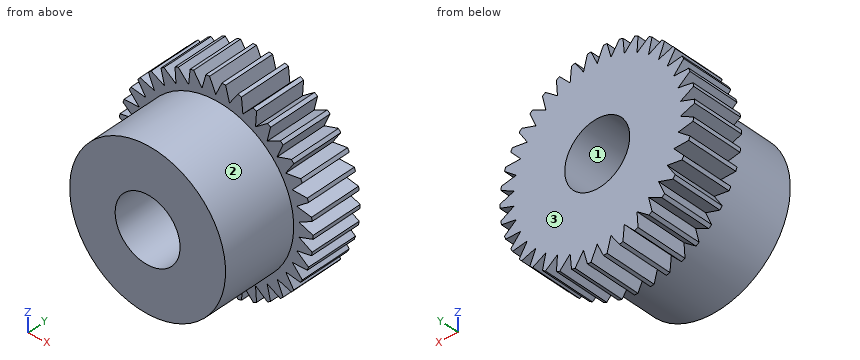
```python
from build123d import *

# Parameters (mm, degrees)
SKETCH_1_R          = 6
EXTRUDE_1_DEPTH     = 5.8
SKETCH_2_R          = 7.5
EXTRUDE_2_DEPTH     = 4
CUT_EXTRUDE_3_DEPTH = 15.440914098
SKETCH_4_R          = 2.5
CUT_EXTRUDE_4_DEPTH = 15.43297622


with BuildPart() as part:
    # Эскиз1 → Вытянуть1 (new body)
    with BuildSketch(Plane(origin=(0, 0, 0), x_dir=(1, 0, 0), z_dir=(0, 1, 0))):
        with Locations(Location((0, 0, 0), (0, 0, 270))):
            Circle(SKETCH_1_R)
    extrude(amount=EXTRUDE_1_DEPTH)

    # Эскиз2 → Вытянуть2 (add)
    with BuildSketch(Plane(origin=(0, 5.8, 0), x_dir=(1, 0, 0), z_dir=(0, 1, 0))):
        with Locations(Location((0, 0, 0), (0, 0, 270))):
            Circle(SKETCH_2_R)
    extrude(amount=EXTRUDE_2_DEPTH)

    # Эскиз3 → Вытянуть3 (cut, through all)
    with BuildSketch(Plane(origin=(0, 9.8, 0), x_dir=(1, 0, 0), z_dir=(0, 1, 0))):
        Polygon((-0.62278932, 7.802539676), (0.62278932, 7.802539676), (0, 6.428342871), align=None)
        Polygon((0.669960535, 7.798630957), (1.898551107, 7.593615451), (1.058070461, 6.340668653), align=None)
        Polygon((1.944435614, 7.581995916), (3.122525368, 7.177557193), (2.087279518, 6.080037523), align=None)
        Polygon((3.165871558, 7.158543791), (4.261325277, 6.565713884), (3.059553031, 5.653558819), align=None)
        Polygon((4.300950779, 6.539825252), (5.283887341, 5.774775016), (3.948369913, 5.072865768), align=None)
        Polygon((5.318711274, 5.742717328), (6.162318733, 4.82631534), (4.729485556, 4.353798163), align=None)
        Polygon((6.19139119, 4.788963046), (6.872658133, 3.746206362), (5.381593163, 3.515970293), align=None)
        Polygon((6.895186095, 3.704578336), (7.395529336, 2.563910641), (5.886904936, 2.582235919), align=None)
        Polygon((7.410898297, 2.519142386), (7.716669776, 1.311678121), (6.231637289, 1.578064881), align=None)
        Polygon((7.724460512, 1.264990798), (7.827319581, 0.023666441), (6.406386821, 0.530848347), align=None)
        Polygon((7.827319581, -0.023666441), (7.724460512, -1.264990798), (6.406386821, -0.530848347), align=None)
        Polygon((7.716669776, -1.311678121), (7.410898297, -2.519142386), (6.231637289, -1.578064881), align=None)
        Polygon((7.395529336, -2.563910641), (6.895186095, -3.704578336), (5.886904936, -2.582235919), align=None)
        Polygon((6.872658133, -3.746206362), (6.19139119, -4.788963046), (5.381593163, -3.515970293), align=None)
        Polygon((6.162318733, -4.82631534), (5.318711274, -5.742717328), (4.729485556, -4.353798163), align=None)
        Polygon((5.283887341, -5.774775016), (4.300950779, -6.539825252), (3.948369913, -5.072865768), align=None)
        Polygon((4.261325277, -6.565713884), (3.165871558, -7.158543791), (3.059553031, -5.653558819), align=None)
        Polygon((3.122525368, -7.177557193), (1.944435614, -7.581995916), (2.087279518, -6.080037523), align=None)
        Polygon((1.898551107, -7.593615451), (0.669960535, -7.798630957), (1.058070461, -6.340668653), align=None)
        Polygon((0.62278932, -7.802539676), (-0.62278932, -7.802539676), (0, -6.428342871), align=None)
        Polygon((-0.669960535, -7.798630957), (-1.898551107, -7.593615451), (-1.058070461, -6.340668653), align=None)
        Polygon((-1.944435614, -7.581995916), (-3.122525368, -7.177557193), (-2.087279518, -6.080037523), align=None)
        Polygon((-3.165871558, -7.158543791), (-4.261325277, -6.565713884), (-3.059553031, -5.653558819), align=None)
        Polygon((-4.300950779, -6.539825252), (-5.283887341, -5.774775016), (-3.948369913, -5.072865768), align=None)
        Polygon((-5.318711274, -5.742717328), (-6.162318733, -4.82631534), (-4.729485556, -4.353798163), align=None)
        Polygon((-6.19139119, -4.788963046), (-6.872658133, -3.746206362), (-5.381593163, -3.515970293), align=None)
        Polygon((-6.895186095, -3.704578336), (-7.395529336, -2.563910641), (-5.886904936, -2.582235919), align=None)
        Polygon((-7.410898297, -2.519142386), (-7.716669776, -1.311678121), (-6.231637289, -1.578064881), align=None)
        Polygon((-7.724460512, -1.264990798), (-7.827319581, -0.023666441), (-6.406386821, -0.530848347), align=None)
        Polygon((-7.827319581, 0.023666441), (-7.724460512, 1.264990798), (-6.406386821, 0.530848347), align=None)
        Polygon((-7.716669776, 1.311678121), (-7.410898297, 2.519142386), (-6.231637289, 1.578064881), align=None)
        Polygon((-7.395529336, 2.563910641), (-6.895186095, 3.704578336), (-5.886904936, 2.582235919), align=None)
        Polygon((-6.872658133, 3.746206362), (-6.19139119, 4.788963046), (-5.381593163, 3.515970293), align=None)
        Polygon((-6.162318733, 4.82631534), (-5.318711274, 5.742717328), (-4.729485556, 4.353798163), align=None)
        Polygon((-5.283887341, 5.774775016), (-4.300950779, 6.539825252), (-3.948369913, 5.072865768), align=None)
        Polygon((-4.261325277, 6.565713884), (-3.165871558, 7.158543791), (-3.059553031, 5.653558819), align=None)
        Polygon((-3.122525368, 7.177557193), (-1.944435614, 7.581995916), (-2.087279518, 6.080037523), align=None)
        Polygon((-1.898551107, 7.593615451), (-0.669960535, 7.798630957), (-1.058070461, 6.340668653), align=None)
    extrude(amount=-CUT_EXTRUDE_3_DEPTH, mode=Mode.SUBTRACT)

    # Эскиз4 → Вытянуть4 (cut, through all)
    with BuildSketch(Plane.XZ):
        with Locations(Location((0, 0, 0), (0, 0, 270))):
            Circle(SKETCH_4_R)
    extrude(amount=-CUT_EXTRUDE_4_DEPTH, mode=Mode.SUBTRACT)


solid = part.part
```
Could you check a few things on this model? Use its own coordinates, in mm. Face numbers are marked on the shaded views. Coordinates: 2 decimals unless noted, no trailing zeros. Loops run counter-clockwise (first coordinate to the right, second up) from the corner with the lowest first, then second, coordinate; pieces in that order, holes last.
1) Imagine slicing it at A-A (z = 0.75). List the corners of the cut face in (x, y) for me, and give its area (3 significant figures).
Reported:
outline: (-6.8, 5.8) - (-5.95, 5.8) - (-5.95, 0) - (-2.38, 0) - (-2.38, 9.8) - (-6.8, 9.8) - close; (2.38, 0) - (5.95, 0) - (5.95, 5.8) - (6.8, 5.8) - (6.8, 9.8) - (2.38, 9.8) - close
area: 76.7 mm2
2) Imagine slicing it at C-C (z = 3). List the corners of the cut face in (x, y) for me.
Reported:
outline: (-6.26, 5.8) - (-5.2, 5.8) - (-5.2, 0) - (5.2, 0) - (5.2, 5.8) - (6.26, 5.8) - (6.26, 9.8) - (-6.26, 9.8) - close
3) Thinking about a two-plate mould opening in Z: for the marked faces 1, 2 and 3, which applies, released by +Z, released by -Z, zero draft, split by the parting line, or undercut?
Reported:
face 1: undercut
face 2: split by the parting line
face 3: zero draft
4) Please list where these lines run through material, in increasing order: line 1 along X through (y, z) = (2.75, 0); line 2 along X through (y, z) = (6, 0); line 3 along Y through (x, z) = (-1.25, -6.25).
Reported:
line 1: x = -6 to -2.5, 2.5 to 6
line 2: x = -7.5 to -2.5, 2.5 to 7.5
line 3: y = 5.8 to 9.8
5) Imagine slicing it at B-B (y = 0.5). List the corners of the cut face in (x, z) for me, and give its area (3 significant figures).
Reported:
outline: circle Ø12 at (0, 0); hole circle Ø5 at (0, 0)
area: 93.5 mm2
